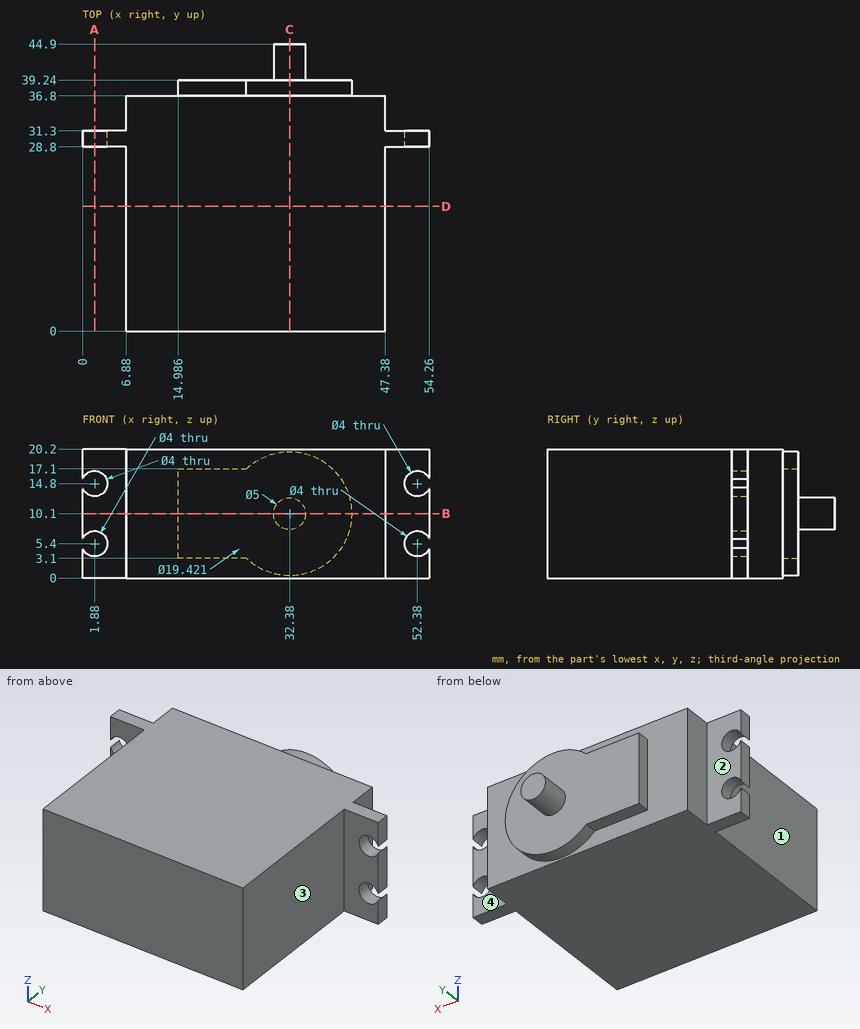
Design review of the part shown in the three views and the two pictorial views. Dimensions are in mm from the part's minimum x, y and z. A direction names the side the tool comes from. Coordinates: 2 decimals unless noted, no trailing zeros. Loops run counter-clockwise (first coordinate to the right, second up) from the corner with the lowest first, then second, coordinate; pieces in that order, holes last. Notation, with made-up numbers: (-29, 14.5) -> (-18, 14.5) arc R25 ccw to (-18, 30.5) -> close; hole circle Ø4 at (47.5, 36.5). An arc over 180 degrees is marked (long way). Answer as CSV lines item,"result".
Item 1: For L1, parallel to Z at x = 52.38, y = 29.55; L2, parallel to Y at x = 34, z = 15.25; L3, parallel to Y at x = 13.5, z = 12.75, list the stretches that pass through material, from the lowest coordinate up.
Results below:
L1,"z = 0 to 3.4, 7.4 to 12.8, 16.8 to 20.2"
L2,"y = 0 to 39.24"
L3,"y = 0 to 36.8"
Item 2: Take a section at C-C, the plane x = 32.38. State the section outline as (y, z) points, and give its area (3 significant figures).
Results below:
outline,"(0, 0) -> (36.8, 0) -> (36.8, 0.39) -> (39.24, 0.39) -> (39.24, 7.6) -> (44.9, 7.6) -> (44.9, 12.6) -> (39.24, 12.6) -> (39.24, 19.81) -> (36.8, 19.81) -> (36.8, 20.2) -> (0, 20.2) -> close"
area,"819 mm2"
Item 3: Take a section at B-B, the plane z = 10.1. State the section outline as (x, y) points.
Results below:
outline,"(0, 28.8) -> (6.88, 28.8) -> (6.88, 0) -> (47.38, 0) -> (47.38, 28.8) -> (54.26, 28.8) -> (54.26, 31.3) -> (47.38, 31.3) -> (47.38, 36.8) -> (42.09, 36.8) -> (42.09, 39.24) -> (34.88, 39.24) -> (34.88, 44.9) -> (29.88, 44.9) -> (29.88, 39.24) -> (14.99, 39.24) -> (14.99, 36.8) -> (6.88, 36.8) -> (6.88, 31.3) -> (0, 31.3) -> close"
Item 4: Insertion check: pin 1 (2 mm diameter, centred on x = 52.5, z = 10, fed in from +Y); pin 2 (3 mm diameter, centred on x = 32.5, z = 4.5, fed in from +Y); pin 3 (1.2 mm diameter, centred on x = 21.5, y = 37.5, fed in from +Z). Each pin has a flat end and moves straight along its axis. Give the tip position at first contact, or say it passes through.
Results below:
pin 1,"stops at y = 31.3"
pin 2,"stops at y = 39.24"
pin 3,"stops at z = 17.1"
Item 5: Take a section at A-A, the plane x = 1.88. State the section outline as (y, z) points.
Results below:
outline,"(28.8, 0) -> (31.3, 0) -> (31.3, 3.4) -> (28.8, 3.4) -> close; (28.8, 7.4) -> (31.3, 7.4) -> (31.3, 12.8) -> (28.8, 12.8) -> close; (28.8, 16.8) -> (31.3, 16.8) -> (31.3, 20.2) -> (28.8, 20.2) -> close"
Item 6: Take a section at D-D, the plane y = 19.5. State the section outline as (x, z) points, and give its area (3 significant figures).
Results below:
outline,"(6.88, 0) -> (47.38, 0) -> (47.38, 20.2) -> (6.88, 20.2) -> close"
area,"818 mm2"
Item 7: Machinability: for the marked faces 1, 2, 3 and 4, which of the approach directions +Z, -Z, +X, -X, +Y, -Y give a long, thin tool a straight path to every point of the face, cutting with its end or side? Answer none if there is none.
Results below:
face 1,"+Z, -Z, -X, -Y"
face 2,"+Z, -Z, -X, +Y"
face 3,"+Z, -Z, +X, -Y"
face 4,"+Z, -Z, +X, +Y"
